Build history of the part. All positions in model axes, mm. Coordinates: 2 decimals unless noted, no trailing zeros. Loops run counter-clockwise (first coordinate to the right, second up) from the corner with the lowest first, then second, coordinate; pieces in that order, holes last.
(1) Wall check: L1, parallel to Y at x = 48, z = -42.5; L2, parallel to Y at x = -29, z = 8.5; L3, parallel to X at y = -19.5, z = 48. Give the ranges that are in metal, low to high.
(2) Flat gauge pins, fed straight in: P1, Ø1, axis at x = 13, z = -46, coming from the +Y side; P2, Ø4, axis at y = -22.5, z = -22, coming from the +X side. Where does each tip first touch, or does it go through?
(3) Slice it at B-B (z = -4.5). Give the cut face in (x, y) (3 decimals).
(4) Slice it at A-A (y = -15.25). Give the cut face in (x, z).
from build123d import *

# Parameters (mm, degrees)
BOSS_EXTRUDE1_DEPTH = 60
FILLET1_R           = 10


with BuildPart() as part:
    # Sketch1 → Boss-Extrude1 (new, symmetric)
    with BuildSketch(Plane.XY):
        with BuildLine():
            Line((52.375, -25.867869753), (52.375, -26.867869753))
            Line((52.375, -26.867869753), (-52.375, -26.867869753))
            Line((-52.375, -26.867869753), (-52.375, -25.867869753))
            ThreePointArc((-52.375, -25.867869753), (0, -11.055071697), (52.375, -25.867869753))
        make_face()
    extrude(amount=BOSS_EXTRUDE1_DEPTH, both=True)

    # Fillet1
    fillet1_edges = [part.edges().sort_by_distance(p)[0] for p in [
        (52.375, -26.367869753, 60),
        (52.375, -26.367869753, -60),
        (-52.375, -26.367869753, -60),
        (-52.375, -26.367869753, 60),
    ]]
    fillet(fillet1_edges, radius=FILLET1_R)


solid = part.part
Response values:
1. L1: y = -26.87 to -23.33
1. L2: y = -26.87 to -15.35
1. L3: x = -40.22 to 40.22
2. P1: stops at y = -11.84
2. P2: stops at x = 50.08
3. outline: (-52.375, -26.868) - (52.375, -26.868) - (52.375, -25.868) arc R100 ccw to (-52.375, -25.868) - close
4. outline: (-28.66, -60) - (28.66, -60) - (28.66, 60) - (-28.66, 60) - close
